from build123d import *

# Parameters (mm, degrees)
BOSS_EXTRUDE1_DEPTH     = 1270
F_1_4_20_TAPPED_HOLE1_D = 5.1054
CUT_EXTRUDE1_DEPTH      = 2.5875


with BuildPart() as part:
    # Sketch2 → Boss-Extrude1 (new body, symmetric)
    with BuildSketch(Plane.XY):
        with BuildLine():
            Line((-12.7, -12.7), (12.7, -12.7))
            Line((12.7, -12.7), (12.7, 12.7))
            Line((12.7, 12.7), (11.90625, 12.7))
            ThreePointArc((11.90625, 12.7), (11.344983992, 12.467516008), (11.1125, 11.90625))
            Line((11.1125, 11.90625), (11.1125, -9.5377))
            ThreePointArc((11.1125, -9.5377), (10.651251759, -10.651251759), (9.5377, -11.1125))
            Line((9.5377, -11.1125), (-11.90625, -11.1125))
            ThreePointArc((-11.90625, -11.1125), (-12.467516008, -11.344983992), (-12.7, -11.90625))
            Line((-12.7, -11.90625), (-12.7, -12.7))
        make_face()
    extrude(amount=BOSS_EXTRUDE1_DEPTH, both=True)

    # 1/4-20 Tapped Hole1 (through all)
    with Locations(Plane(origin=(0, -11.1125, 0), x_dir=(1, 0, 0), z_dir=(0, 1, 0))):
        with Locations((-1.5875, -1017.524), (-1.5875, -561.848), (-1.5875, 349.504), (-1.5875, -106.172)):
            Hole(F_1_4_20_TAPPED_HOLE1_D / 2)

    # Sketch5 → Cut-Extrude1 (cut, through all)
    with BuildSketch(Plane(origin=(0, -11.1125, 0), x_dir=(1, 0, 0), z_dir=(0, 1, 0))):
        with BuildLine():
            Line((1.4605, -1057.275), (1.4605, -1076.325))
            ThreePointArc((1.4605, -1076.325), (-1.5875, -1079.373), (-4.6355, -1076.325))
            Line((-4.6355, -1076.325), (-4.6355, -1057.275))
            ThreePointArc((-4.6355, -1057.275), (-1.5875, -1054.227), (1.4605, -1057.275))
        make_face()
        with BuildLine():
            Line((1.4605, -641.35), (1.4605, -660.4))
            ThreePointArc((1.4605, -660.4), (-1.5875, -663.448), (-4.6355, -660.4))
            Line((-4.6355, -660.4), (-4.6355, -641.35))
            ThreePointArc((-4.6355, -641.35), (-1.5875, -638.302), (1.4605, -641.35))
        make_face()
        with BuildLine():
            Line((1.4605, 317.5), (1.4605, 336.55))
            ThreePointArc((1.4605, 336.55), (-1.5875, 339.598), (-4.6355, 336.55))
            Line((-4.6355, 336.55), (-4.6355, 317.5))
            ThreePointArc((-4.6355, 317.5), (-1.5875, 314.452), (1.4605, 317.5))
        make_face()
        with BuildLine():
            Line((1.4605, 717.55), (1.4605, 1092.2))
            ThreePointArc((1.4605, 1092.2), (-1.5875, 1095.248), (-4.6355, 1092.2))
            Line((-4.6355, 1092.2), (-4.6355, 717.55))
            ThreePointArc((-4.6355, 717.55), (-1.5875, 714.502), (1.4605, 717.55))
        make_face()
    extrude(amount=-CUT_EXTRUDE1_DEPTH, mode=Mode.SUBTRACT)


solid = part.part
The listing builds one solid part. Answer for the finished solid, in the listing's coordinates (mm). Coordinates: 2 decimals unless noted, no trailing zeros. Write each loop counter-clockwise with the first axis right and the second up, starting at its lowest first coordinate (ties: lowest second). Pieces come first, ordered by that corner, then holes. Notation, with made-up numbers: M -37.75,10.5 L -33.75,10.5 A20 cw -33.75,42.5 Z; hole C 72,-28.5 d8. An arc over 180 degrees is marked long. Put each result on its own line as item: value. Start each with the question number.
1. Flat-ended cylindrical pins translate along their axes: P1, Ø6.5, axis at y = 1.5, z = -66, coming from the -X side; P2, Ø6.5, axis at x = -1.59, z = 561.85, coming from the +Y side; P3, Ø8, axis at y = -6.5, z = -922, coming from the -X side. Find the tip coordinate at first contact, or state that the pin passes through.
2. A cutting plane is placed at B-B on y = 5.75. Write down the section's boundary in (x, z), then the cut area to 3 significant figures.
3. A cutting plane is placed at A-A on z = 775.5. Write down the section's boundary in (x, y).
4. Consider line 1 (Y direction, x = 1.25, z = 821.5); line 2 (X direction, y = 1.5, z = -501.5); line 3 (Y direction, x = 11.5, z = -300). Determine where each line is inside the solid, lowest interval first. Write a range as from..to.
Resolved:
1. P1: stops at x = 11.11
1. P2: stops at y = -11.11
1. P3: stops at x = 10.78
2. outline: M 11.11,-1270 L 12.7,-1270 L 12.7,1270 L 11.11,1270 Z
2. area: 4,030 mm2
3. outline: M -12.7,-12.7 L 12.7,-12.7 L 12.7,12.7 L 11.91,12.7 A0.79 ccw 11.11,11.91 L 11.11,-9.54 A1.57 cw 9.54,-11.11 L -11.91,-11.11 A0.79 ccw -12.7,-11.91 Z
4. line 1: y = -12.7..-11.11
4. line 2: x = 11.11..12.7
4. line 3: y = -12.7..12.59
